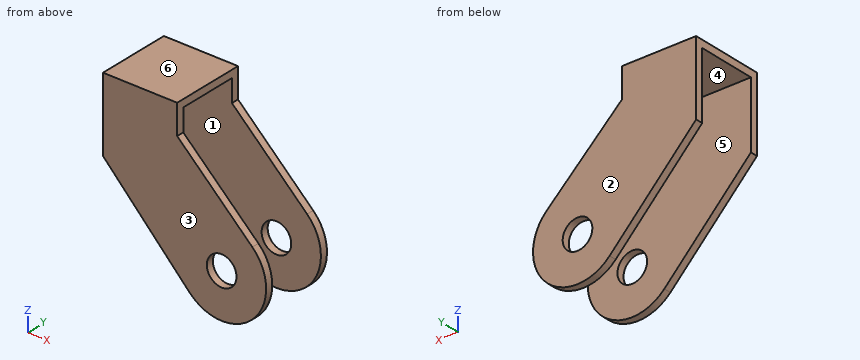
```python
from build123d import *

# Parameters (mm, degrees)
F0_R     = 20
F1_DEPTH = 10
F4_W     = 100
F4_H     = 10
F5_DEPTH = 80


with BuildPart() as f1:
    # F0 (on Front) → F1 (new body)
    with BuildSketch(Plane.XZ):
        with BuildLine():
            Line((100, 0), (0, 0))
            Line((0, 0), (0, -100))
            Line((0, -100), (116.7215506805, -221.5568986391))
            ThreePointArc((116.7215506805, -221.5568986391), (202.5131933075, -222.3394425423), (201.3793103448, -136.5517241379))
            Line((201.3793103448, -136.5517241379), (100, -40))
            Line((100, -40), (100, 0))
        make_face()
        with Locations((160, -180)):
            Circle(F0_R, mode=Mode.SUBTRACT)
    extrude(amount=-F1_DEPTH)


with BuildPart() as f3_1:
    # F3: instance of F1
    add(f1.part.mirror(Plane.XZ.offset(-50)))


with BuildPart() as f1_1:
    add(f1.part)

    add(f3_1.part)  # F5 merges F3_1
    # F4 (on face) → F5 (join, through all)
    with BuildSketch(Plane.XZ.offset(-90)):
        with Locations((50, -5)):
            Rectangle(F4_W, F4_H)
    extrude(amount=F5_DEPTH)


solid = f1_1.part
```
Geometry: final body of the model. Coordinates: model frame, mm. Face numbers are marked on the shaded views. A direction names the side the tool comes from. Round coordinates to 2 decimals unless told otherwise and drop trailing zeros. Write each loop counter-clockwise with the first axis right and the second up, starting at its lowest first coordinate (ties: lowest second). Pieces come first, ordered by that corner, then holes. Notation, with made-up numbers: M 30,76.25 L 42,76.25 A9 cw 42,88.25 Z; hole C 54,-9 d7. An arc over 180 degrees is marked long. Answer in a Markdown table with one row per item. Add a question column.
(1) Cut plane D-D, the plane x = 160. Return the cut outline in (y, z).
(2) Ray query, L1, parallel to Y at x = 164.5, z = -143; L2, parallel to Z at x = 160, y = 3; L3, parallel to X at y = 96, z = -10. Return the intervals inside material, ascending.
(3) Cut plane A-A, the plane z = -49. Return the cut outline in (x, y).
(4) Cut plane C-C, the plane z = -180. Return the cut outline in (x, y).
(5) Cut plane B-B, the plane x = 109.5. Return the cut outline in (y, z).
(6) Draft query along Y for the marked faces 1, 2, 3 and 4. Return one class per face: pulls with the +Y half, pulls with the -Y half, needs draft (parallel to the pull), parting line crosses it, or undercut.
(7) Reachability of the marked faces 5 and 6 from +Z, -Z, +X, -X, +Y, -Y: full face, straight path, thin tool, end or side. Return the list, or none.
Established:
| question | item | result |
|---|---|---|
| 1 | outline | M 0,-240 L 10,-240 L 10,-200 L 0,-200 Z; M 0,-160 L 10,-160 L 10,-97.14 L 0,-97.14 Z; M 90,-240 L 100,-240 L 100,-200 L 90,-200 Z; M 90,-160 L 100,-160 L 100,-97.14 L 90,-97.14 Z |
| 2 | L1 | 0 to 10, 90 to 100 |
| 2 | L2 | -240 to -200, -160 to -97.14 |
| 2 | L3 | 0 to 100 |
| 3 | outline | M 0,0 L 109.45,0 L 109.45,10 L 0,10 Z; M 0,90 L 109.45,90 L 109.45,100 L 0,100 Z |
| 4 | outline | M 76.82,0 L 140,0 L 140,10 L 76.82,10 Z; M 76.82,90 L 140,90 L 140,100 L 76.82,100 Z; M 180,0 L 220,0 L 220,10 L 180,10 Z; M 180,90 L 220,90 L 220,100 L 180,100 Z |
| 5 | outline | M 0,-214.04 L 10,-214.04 L 10,-49.05 L 0,-49.05 Z; M 90,-214.04 L 100,-214.04 L 100,-49.05 L 90,-49.05 Z |
| 6 | face 1 | undercut |
| 6 | face 2 | pulls with the +Y half |
| 6 | face 3 | pulls with the -Y half |
| 6 | face 4 | undercut |
| 7 | face 5 | -Z, +X, -X |
| 7 | face 6 | +Z, +X, -X, +Y, -Y |
